Could you check a few things on this model? Use its own coordinates, in mm. A direction names the side the tool comes from. Give positions to 0.01 mm unless a question says otherwise; leave off trailing zeros. Write each loop counter-clockwise with the first axis right and the second up, starting at its lowest first coordinate (ties: lowest second). Pieces come first, ordered by that corner, then holes. Notation, with made-up numbers: (-39.5, 10) - (1.5, 10) arc R19 ccw to (1.5, 38) - close; hole circle Ø9 at (23, 31.5). An arc over 180 degrees is marked (long way). Use one line per item in the form item = value.
```python
from build123d import *

# Parameters (mm, degrees)
SKETCH4_R           = 3.69
BOSS_EXTRUDE2_DEPTH = 13.7
SKETCH5_R           = 2.75
CUT_EXTRUDE2_DEPTH  = 1.5
CUT_EXTRUDE3_DEPTH  = 7.2
SKETCH7_W           = 1.9
SKETCH7_H           = 1.5
SKETCH7_H_2         = 1.9
SKETCH7_W_2         = 1.5
CUT_EXTRUDE5_DEPTH  = 5
FILLET1_R           = 0.75
FILLET2_R           = 0.75
FILLET3_R           = 0.75
FILLET4_R           = 0.75


with BuildPart() as part:
    # Sketch4 → Boss-Extrude2 (new body)
    with BuildSketch(Plane(origin=(0, 0, 0), x_dir=(1, 0, 0), z_dir=(0, 1, 0))):
        with Locations((-30.556065381, -14.685726519)):
            Circle(SKETCH4_R)
    extrude(amount=BOSS_EXTRUDE2_DEPTH)

    # Sketch5 → Cut-Extrude2 (cut)
    with BuildSketch(Plane(origin=(0, 13.7, 0), x_dir=(1, 0, 0), z_dir=(0, 1, 0))):
        with Locations((-30.556065381, -14.685726519)):
            Circle(SKETCH5_R)
    extrude(amount=-CUT_EXTRUDE2_DEPTH, mode=Mode.SUBTRACT)

    # Sketch6 → Cut-Extrude3 (cut)
    with BuildSketch(Plane(origin=(0, 12.2, 0), x_dir=(1, 0, 0), z_dir=(0, 1, 0))):
        with BuildLine():
            ThreePointArc((-32.456065381, -16.673816054), (-30.556065381, -17.435726519), (-28.656065381, -16.673816054))
            Line((-28.656065381, -16.673816054), (-28.656065381, -12.697636984))
            ThreePointArc((-28.656065381, -12.697636984), (-30.556065381, -11.935726519), (-32.456065381, -12.697636984))
            Line((-32.456065381, -12.697636984), (-32.456065381, -16.673816054))
        make_face()
    extrude(amount=-CUT_EXTRUDE3_DEPTH, mode=Mode.SUBTRACT)

    # Sketch7 → Cut-Extrude5 (cut)
    with BuildSketch(Plane(origin=(0, 0, 0), x_dir=(-1, 0, 0), z_dir=(0, -1, 0))):
        with Locations((30.556065381, -16.385726519)):
            Rectangle(SKETCH7_W, SKETCH7_H)
        with Locations((30.556065381, -14.685726519)):
            Rectangle(SKETCH7_W, SKETCH7_H_2)
        with Locations((28.856065381, -14.685726519)):
            Rectangle(SKETCH7_W_2, SKETCH7_H_2)
        with Locations((32.256065381, -14.685726519)):
            Rectangle(SKETCH7_W_2, SKETCH7_H_2)
        with Locations((30.556065381, -12.985726519)):
            Rectangle(SKETCH7_W, SKETCH7_H)
    extrude(amount=-CUT_EXTRUDE5_DEPTH, mode=Mode.SUBTRACT)

    # Fillet1
    fillet1_edges = [part.edges().sort_by_distance(p)[0] for p in [
        (-31.506065381, 2.5, 15.635726519),
    ]]
    fillet(fillet1_edges, radius=FILLET1_R)

    # Fillet2
    fillet2_edges = [part.edges().sort_by_distance(p)[0] for p in [
        (-29.606065381, 2.5, 13.735726519),
    ]]
    fillet(fillet2_edges, radius=FILLET2_R)

    # Fillet3
    fillet3_edges = [part.edges().sort_by_distance(p)[0] for p in [
        (-29.606065381, 2.5, 15.635726519),
    ]]
    fillet(fillet3_edges, radius=FILLET3_R)

    # Fillet4
    fillet4_edges = [part.edges().sort_by_distance(p)[0] for p in [
        (-31.506065381, 2.5, 13.735726519),
    ]]
    fillet(fillet4_edges, radius=FILLET4_R)


solid = part.part
```
1. Imagine slicing it at A-A, the plane z = 12.5. List the corners of the cut face in (x, y) for me.
Response values:
outline = (-33.53, 0) - (-31.51, 0) - (-31.51, 5) - (-32.22, 5) - (-32.22, 13.7) - (-33.53, 13.7) - close; (-29.61, 0) - (-27.58, 0) - (-27.58, 13.7) - (-28.89, 13.7) - (-28.89, 5) - (-29.61, 5) - close
2. Imagine slicing it at C-C, the plane x = -28.25. List the corners of the cut face in (y, z) for me, and give its area (3 significant figures).
Response values:
outline = (0, 11.81) - (13.7, 11.81) - (13.7, 13.19) - (12.2, 13.19) - (12.2, 16.18) - (13.7, 16.18) - (13.7, 17.57) - (0, 17.57) - (0, 15.64) - (5, 15.64) - (5, 13.74) - (0, 13.74) - close
area = 64.9 mm²
3. Imagine slicing it at B-B, the plane x = -32. List the corners of the cut face in (y, z) for me.
Response values:
outline = (0, 11.29) - (13.7, 11.29) - (13.7, 12.35) - (5, 12.35) - (5, 13.69) - (0, 13.69) - close; (0, 15.68) - (5, 15.68) - (5, 17.03) - (13.7, 17.03) - (13.7, 18.08) - (0, 18.08) - close
4. Imagine slicing it at D-D, the plane y = 3.5. List the corners of the cut face in (x, z) for me, and give its area (3 significant figures).
Response values:
outline = circle Ø7.38 at (-30.56, 14.69); hole (-33.01, 13.74) - (-32.26, 13.74) arc R0.75 cw to (-31.51, 12.99) - (-31.51, 12.24) - (-29.61, 12.24) - (-29.61, 12.99) arc R0.75 cw to (-28.86, 13.74) - (-28.11, 13.74) - (-28.11, 15.64) - (-28.86, 15.64) arc R0.75 cw to (-29.61, 16.39) - (-29.61, 17.14) - (-31.51, 17.14) - (-31.51, 16.39) arc R0.75 cw to (-32.26, 15.64) - (-33.01, 15.64) - close
area = 27.3 mm²
5. Which directions (+Z, -Z, +X, -X, +Y, -Y) give clear straight access to the entire face, cutting with the end or side of a thin tool? Please do faces 1 (the face through (-28, 12.2, 15)), 2 (the face through (-31, 2, 17.136)), 3 (the face through (-28.106, 2, 15)).
Response values:
face_1 = +Y
face_2 = +Y, -Y
face_3 = -Y
6. If I drill on line 1 (X direction, y = 11.75, z = 14.75); line 2 (Z direction, x = -28.75, y = 12.25); line 3 (Z direction, x = -29, y = 1), over which ranges is the centre line in solid material (lowest first)? Write a range as from..to.
Response values:
line_1 = -34.25..-32.46, -28.66..-26.87
line_2 = 11.47..12.61, 16.76..17.9
line_3 = 11.34..13.72, 15.65..18.03
7. For pin 1 (2 mm diameter, centred on x = -28, y = 10, fed in from -Z); pin 2 (0.8 mm diameter, centred on y = 2.5, z = 16.5, fed in from +X); pin 3 (2 mm diameter, centred on y = 7.5, z = 17.5, fed in from +X), each with a flat end and sliding along its axis, tell me the tip position at first contact or that it passes through.
Response values:
pin_1 = 11.34
pin_2 = -27.15
pin_3 = -27.34
8. If we mould it in two halves opening along X, with no side actions, what happens to faces 4 (the face through (-31, 2, 12.236)), 5 (the face through (-32, 0, 13)), 6 (the face through (-27.036, 6.754, 13.577))? For each: pulls with the +X half, pulls with the -X half, needs draft (parallel to the pull), parting line crosses it, or undercut.
Response values:
face_4 = undercut
face_5 = needs draft
face_6 = parting line crosses it
